Build history of the part. All positions in model axes, mm. Face numbers are marked on the shaded views. A direction names the side the tool comes from. Round coordinates to 2 decimals unless told otherwise and drop trailing zeros. Order: outer loops, then holes, each group sorted by start corner. A loop starts at its lowest first (then second) coordinate and runs counter-clockwise, first axis right, second up. Notation, with made-up numbers: (-34.75, 52.25) -> (-11.75, 52.25) arc R20 ccw to (-11.75, 60.25) -> close; hole circle Ø10 at (18.25, 51.25). An arc over 180 degrees is marked (long way). Use a Markdown table: item, result. Add a question column.
Item 1: Slice it at D-D, the plane z = 17.25. Give the cut face in (x, y), plus the area to 3 significant figures.
Item 2: Probe L1, parallel to Y at x = 11, z = 14; L2, parallel to X at y = 12, z = 9; L3, parallel to Z at x = -10, y = 4. List the from-to ranges inside material, lowest first.
Item 3: Slice it at B-B, the plane x = -15.5. Give the cut face in (y, z).
Item 4: 3-axis set-ups, long thin cutter, end or side, ignore diameter. For the marked faces 1, 2 and 3: which of +Z, -Z, +X, -X, +Y, -Y reach the whole face in a straight line?
Item 5: Pin check, flat tips, straight feed: pin 1 (17 mm diameter, centred on x = 1, y = -5, fed in from +Z); pin 2 (2 mm diameter, centred on x = -14, y = 7, fed in from -Z). Stop position of each tip, or through.
Item 6: Slice it at A-A, the plane z = 1.5. Give the cut face in (x, y).
Item 7: Two-plate mould, pull along X, no slides. Class the marked faces 4, 5 and 6: released by +X, released by -X, zero draft, split by the parting line, or undercut.
Item 8: Slice it at C-C, the plane y = -4. Give the cut face in (x, z), plus the area to 3 significant figures.
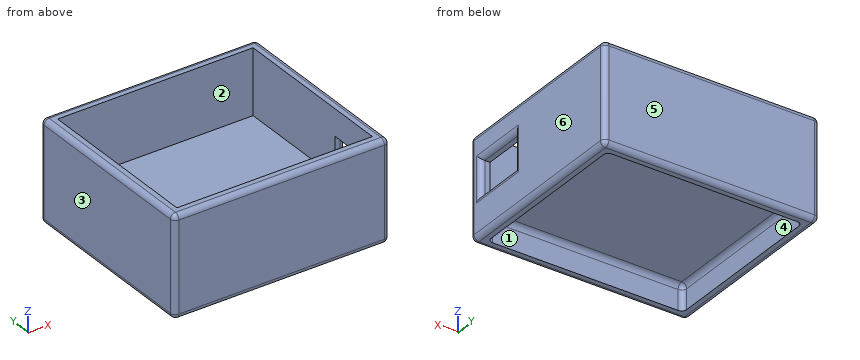
from build123d import *

# Parameters (mm, degrees)
SKETCH_W        = 43
SKETCH_H        = 38
PAD_DEPTH       = 20
SKETCH002_W     = 39
SKETCH002_H     = 34
POCKET001_DEPTH = 5
SKETCH003_W     = 39
SKETCH003_H     = 34
POCKET_DEPTH    = 13
FILLET_R        = 1
FILLET001_R     = 1
FILLET002_R     = 1
FILLET003_R     = 1
FILLET004_R     = 1
FILLET005_R     = 1
FILLET006_R     = 1
FILLET007_R     = 1
FILLET008_R     = 1
FILLET009_R     = 1
SKETCH005_W     = 10
SKETCH005_H     = 7
POCKET002_DEPTH = 5
FILLET010_R     = 1


with BuildPart() as part:
    # Sketch → Pad (new body)
    with BuildSketch(Plane.XY):
        Rectangle(SKETCH_W, SKETCH_H)
    extrude(amount=PAD_DEPTH)

    # Sketch002 → Pocket001 (cut)
    with BuildSketch(Plane(origin=(0, 0, 0), x_dir=(1, 0, 0), z_dir=(0, 0, -1))):
        Rectangle(SKETCH002_W, SKETCH002_H)
    extrude(amount=-POCKET001_DEPTH, mode=Mode.SUBTRACT)

    # Sketch003 (on Face5 of Pocket001) → Pocket (cut)
    with BuildSketch(Plane.XY.offset(20)):
        Rectangle(SKETCH003_W, SKETCH003_H)
    extrude(amount=-POCKET_DEPTH, mode=Mode.SUBTRACT)

    # Fillet
    fillet_edges = [part.edges().sort_by_distance(p)[0] for p in [
        (19.5, 0, 5),
    ]]
    fillet(fillet_edges, radius=FILLET_R)

    # Fillet001
    fillet001_edges = [part.edges().sort_by_distance(p)[0] for p in [
        (-0.5, -17, 5),
    ]]
    fillet(fillet001_edges, radius=FILLET001_R)

    # Fillet002
    fillet002_edges = [part.edges().sort_by_distance(p)[0] for p in [
        (-0.5, 17, 5),
    ]]
    fillet(fillet002_edges, radius=FILLET002_R)

    # Fillet003
    fillet003_edges = [part.edges().sort_by_distance(p)[0] for p in [
        (-19.5, 0, 5),
    ]]
    fillet(fillet003_edges, radius=FILLET003_R)

    # Fillet004
    fillet004_edges = [part.edges().sort_by_distance(p)[0] for p in [
        (-21.5, -19, 10),
    ]]
    fillet(fillet004_edges, radius=FILLET004_R)

    # Fillet005
    fillet005_edges = [part.edges().sort_by_distance(p)[0] for p in [
        (-21.5, 19, 10),
    ]]
    fillet(fillet005_edges, radius=FILLET005_R)

    # Fillet006
    fillet006_edges = [part.edges().sort_by_distance(p)[0] for p in [
        (21.5, 19, 10),
    ]]
    fillet(fillet006_edges, radius=FILLET006_R)

    # Fillet007
    fillet007_edges = [part.edges().sort_by_distance(p)[0] for p in [
        (21.5, -19, 10),
    ]]
    fillet(fillet007_edges, radius=FILLET007_R)

    # Fillet008
    fillet008_edges = [part.edges().sort_by_distance(p)[0] for p in [
        (21.5, 0, 0),
    ]]
    fillet(fillet008_edges, radius=FILLET008_R)

    # Fillet009
    fillet009_edges = [part.edges().sort_by_distance(p)[0] for p in [
        (21.5, 0, 20),
    ]]
    fillet(fillet009_edges, radius=FILLET009_R)

    # Sketch005 (on Face20 of Fillet009) → Pocket002 (cut)
    with BuildSketch(Plane(origin=(19.5, 0, 0), x_dir=(0, -1, 0), z_dir=(-1, 0, 0))):
        with Locations((11.312831, 11.218941)):
            Rectangle(SKETCH005_W, SKETCH005_H)
    extrude(amount=-POCKET002_DEPTH, mode=Mode.SUBTRACT)

    # Fillet010
    fillet010_edges = [part.edges().sort_by_distance(p)[0] for p in [
        (21.5, -11.312831, 7.718941),
        (21.5, -16.312831, 11.218941),
        (21.5, -11.312831, 14.718941),
        (21.5, -6.312831, 11.218941),
    ]]
    fillet(fillet010_edges, radius=FILLET010_R)


solid = part.part
Check sheet entries:
| question | item | result |
|---|---|---|
| 1 | outline | (-21.5, -18) arc R1 ccw to (-20.5, -19) -> (20.5, -19) arc R1 ccw to (21.5, -18) -> (21.5, 18) arc R1 ccw to (20.5, 19) -> (-20.5, 19) arc R1 ccw to (-21.5, 18) -> close; hole (-19.5, -17) -> (19.5, -17) -> (19.5, 17) -> (-19.5, 17) -> close |
| 1 | area | 307 mm2 |
| 2 | L1 | -19 to -17, 17 to 19 |
| 2 | L2 | -21.5 to -19.5, 19.5 to 21.5 |
| 2 | L3 | 5 to 7 |
| 3 | outline | (-19, 1) arc R1 ccw to (-18, 0) -> (-17, 0) -> (-17, 4) arc R1 cw to (-16, 5) -> (16, 5) arc R1 cw to (17, 4) -> (17, 0) -> (18, 0) arc R1 ccw to (19, 1) -> (19, 19) arc R1 ccw to (18, 20) -> (17, 20) -> (17, 7) -> (-17, 7) -> (-17, 20) -> (-18, 20) arc R1 ccw to (-19, 19) -> close |
| 4 | face 1 | -Z |
| 4 | face 2 | +Z |
| 4 | face 3 | +Z, -Z, -X, +Y, -Y |
| 5 | pin 1 | z = 7 |
| 5 | pin 2 | z = 5 |
| 6 | outline | (-21.5, -18) arc R1 ccw to (-20.5, -19) -> (20.5, -19) arc R1 ccw to (21.5, -18) -> (21.5, 18) arc R1 ccw to (20.5, 19) -> (-20.5, 19) arc R1 ccw to (-21.5, 18) -> close; hole (-19.5, -16) arc R1 ccw to (-18.5, -17) -> (18.5, -17) arc R1 ccw to (19.5, -16) -> (19.5, 16) arc R1 ccw to (18.5, 17) -> (-18.5, 17) arc R1 ccw to (-19.5, 16) -> close |
| 7 | face 4 | undercut |
| 7 | face 5 | zero draft |
| 7 | face 6 | released by +X |
| 8 | outline | (-21.5, 1) arc R1 ccw to (-20.5, 0) -> (-19.5, 0) -> (-19.5, 4) arc R1 cw to (-18.5, 5) -> (18.5, 5) arc R1 cw to (19.5, 4) -> (19.5, 0) -> (20.5, 0) arc R1 ccw to (21.5, 1) -> (21.5, 19) arc R1 ccw to (20.5, 20) -> (19.5, 20) -> (19.5, 7) -> (-19.5, 7) -> (-19.5, 20) -> (-20.5, 20) arc R1 ccw to (-21.5, 19) -> close |
| 8 | area | 158 mm2 |
